from build123d import *
from build123d.topology import SkipClean

# Parameters (mm, degrees)
SKETCH1_R                = 9.3
SKETCH1_R_2              = 6.15
BOSS_EXTRUDE1_DEPTH      = 12.2
BOSS_EXTRUDE2_START      = 4
SKETCH2_R                = 9.3
SKETCH2_R_2              = 6.15
BOSS_EXTRUDE2_DEPTH      = 12
BOSS_EXTRUDE3_DEPTH      = 10
BOSS_EXTRUDE3_DEPTH_BACK = 6
SKETCH3_R                = 13.3
SKETCH3_R_2              = 12.3
SKETCH4_R                = 13.3
SKETCH4_R_2              = 9.3
BOSS_EXTRUDE4_DEPTH      = 2
CUT_EXTRUDE1_START       = -6
CUT_EXTRUDE1_DEPTH       = 6
CUT_EXTRUDE2_START       = -16
CUT_EXTRUDE2_DEPTH       = 6
BOSS_EXTRUDE5_START      = 4
SKETCH7_R                = 9.3
BOSS_EXTRUDE5_DEPTH      = 4
BOSS_EXTRUDE6_START      = 2
SKETCH8_R                = 13.3
SKETCH8_R_2              = 9.3
BOSS_EXTRUDE6_DEPTH      = 2
SKETCH9_R                = 9.3
SKETCH9_R_2              = 6.15
BOSS_EXTRUDE7_DEPTH      = 4
FILLET1_R                = 4
FILLET2_R                = 4
FILLET3_R                = 2
FILLET4_R                = 2
FILLET5_R                = 2


# Some blends are built 0.0001 mm under size
with BuildPart() as part:
    # Sketch1 → Boss-Extrude1 (new body)
    with BuildSketch(Plane(origin=(0, 0, 0), x_dir=(1, 0, 0), z_dir=(0, 1, 0))):
        with Locations(Location((0, 0, 0), (0, 0, 270))):
            Circle(SKETCH1_R)
        with Locations(Location((0, 0, 0), (0, 0, 270))):
            Circle(SKETCH1_R_2, mode=Mode.SUBTRACT)
    extrude(amount=BOSS_EXTRUDE1_DEPTH)

    # Sketch5 → Cut-Extrude1 (cut)
    with BuildSketch(Plane.XZ.offset(CUT_EXTRUDE1_START)):
        with BuildLine():
            Line((9.01494402, 2.284903569), (5.709791212, 2.284903569))
            ThreePointArc((5.709791212, 2.284903569), (6.038945105, 1.163461226), (6.15, 0))
            ThreePointArc((6.15, 0), (6.088696755, -0.866182327), (5.906009163, -1.715096431))
            Line((5.906009163, -1.715096431), (9.140483807, -1.715096431))
            ThreePointArc((9.140483807, -1.715096431), (9.260035081, -0.861249265), (9.3, 0))
            ThreePointArc((9.3, 0), (9.228460852, 1.151308085), (9.01494402, 2.284903569))
        make_face()
        with BuildLine():
            ThreePointArc((2, -5.815711478), (0, -6.15), (-2, -5.815711478))
            Line((-2, -5.815711478), (-2, -9.082400564))
            ThreePointArc((-2, -9.082400564), (0, -9.3), (2, -9.082400564))
            Line((2, -9.082400564), (2, -5.815711478))
        make_face()
        with BuildLine():
            ThreePointArc((-5.815711478, -2), (-6.15, 0), (-5.815711478, 2))
            Line((-5.815711478, 2), (-9.082400564, 2))
            ThreePointArc((-9.082400564, 2), (-9.3, 0), (-9.082400564, -2))
            Line((-9.082400564, -2), (-5.815711478, -2))
        make_face()
        with BuildLine():
            ThreePointArc((-2, 5.815711478), (0, 6.15), (2, 5.815711478))
            Line((2, 5.815711478), (2, 9.082400564))
            ThreePointArc((2, 9.082400564), (0, 9.3), (-2, 9.082400564))
            Line((-2, 9.082400564), (-2, 5.815711478))
        make_face()
    extrude(amount=-CUT_EXTRUDE1_DEPTH, mode=Mode.SUBTRACT)



with BuildPart() as body_2:
    # Sketch2 → Boss-Extrude2 (new body)
    with BuildSketch(Plane(origin=(0, 12.2, 0), x_dir=(1, 0, 0), z_dir=(0, 1, 0)).offset(BOSS_EXTRUDE2_START)):
        with Locations(Location((0, 0, 0), (0, 0, 270))):
            Circle(SKETCH2_R)
        with Locations(Location((0, 0, 0), (0, 0, 270))):
            Circle(SKETCH2_R_2, mode=Mode.SUBTRACT)
    extrude(amount=BOSS_EXTRUDE2_DEPTH)



with BuildPart() as body_3:
    # Sketch3 → Boss-Extrude3 (new, two sides: drawn at the far end of the back side and taken through both)
    with BuildSketch(Plane(origin=(0, 12.2, 0), x_dir=(1, 0, 0), z_dir=(0, 1, 0)).offset(-BOSS_EXTRUDE3_DEPTH_BACK)):
        with Locations(Location((0, 0, 0), (0, 0, 270))):
            Circle(SKETCH3_R)
        with Locations(Location((0, 0, 0), (0, 0, 270))):
            Circle(SKETCH3_R_2, mode=Mode.SUBTRACT)
    extrude(amount=BOSS_EXTRUDE3_DEPTH + BOSS_EXTRUDE3_DEPTH_BACK)


with BuildPart() as body_2_1:
    add(body_2.part)

    add(body_3.part)  # Boss-Extrude4 merges body 3
    # Sketch4 → Boss-Extrude4 (add)
    with BuildSketch(Plane(origin=(0, 22.2, 0), x_dir=(1, 0, 0), z_dir=(0, 1, 0))):
        with Locations(Location((0, 0, 0), (0, 0, 270))):
            Circle(SKETCH4_R)
        with Locations(Location((0, 0, 0), (0, 0, 270))):
            Circle(SKETCH4_R_2, mode=Mode.SUBTRACT)
    extrude(amount=BOSS_EXTRUDE4_DEPTH)

    # Sketch6 → Cut-Extrude2 (cut)
    with BuildSketch(Plane.XZ.offset(CUT_EXTRUDE2_START)):
        with BuildLine():
            ThreePointArc((2, -5.815711478), (0, -6.15), (-2, -5.815711478))
            Line((-2, -5.815711478), (-2, -9.082400564))
            ThreePointArc((-2, -9.082400564), (0, -9.3), (2, -9.082400564))
            Line((2, -9.082400564), (2, -5.815711478))
        make_face()
        with BuildLine():
            Line((-9.082400564, -2), (-5.815711478, -2))
            ThreePointArc((-5.815711478, -2), (-6.15, 0), (-5.815711478, 2))
            Line((-5.815711478, 2), (-9.082400564, 2))
            ThreePointArc((-9.082400564, 2), (-9.3, 0), (-9.082400564, -2))
        make_face()
        with BuildLine():
            Line((-2, 9.082400564), (-2, 5.815711478))
            ThreePointArc((-2, 5.815711478), (0, 6.15), (2, 5.815711478))
            Line((2, 5.815711478), (2, 9.082400564))
            ThreePointArc((2, 9.082400564), (0, 9.3), (-2, 9.082400564))
        make_face()
        with BuildLine():
            Line((9.082400564, 2), (5.815711478, 2))
            ThreePointArc((5.815711478, 2), (6.06585219, 1.01387238), (6.15, 0))
            ThreePointArc((6.15, 0), (6.06585219, -1.01387238), (5.815711478, -2))
            Line((5.815711478, -2), (9.082400564, -2))
            ThreePointArc((9.082400564, -2), (9.245440099, -1.005901277), (9.3, 0))
            ThreePointArc((9.3, 0), (9.245440099, 1.005901277), (9.082400564, 2))
        make_face()
    extrude(amount=-CUT_EXTRUDE2_DEPTH, mode=Mode.SUBTRACT)


with BuildPart() as part_1:
    add(part.part)

    add(body_2_1.part)  # Boss-Extrude5 merges body 2
    # Sketch7 → Boss-Extrude5 (add)
    with BuildSketch(Plane.XZ.offset(-16.2).offset(BOSS_EXTRUDE5_START)):
        with Locations(Location((0, 0, 0), (0, 0, 90))):
            Circle(SKETCH7_R)
    extrude(amount=-BOSS_EXTRUDE5_DEPTH)

    # Sketch8 → Boss-Extrude6 (add)
    with BuildSketch(Plane.XZ.offset(-6.2).offset(BOSS_EXTRUDE6_START)):
        with Locations(Location((0, 0, 0), (0, 0, 270))):
            Circle(SKETCH8_R)
        with Locations(Location((0, 0, 0), (0, 0, 282.418681506))):
            Circle(SKETCH8_R_2, mode=Mode.SUBTRACT)
    extrude(amount=-BOSS_EXTRUDE6_DEPTH)

    # Sketch9 → Boss-Extrude7 (add)
    with SkipClean():  # the faces are left unmerged after this step: merging them gives an invalid solid
        with BuildSketch(Plane(origin=(0, 28.2, 0), x_dir=(1, 0, 0), z_dir=(0, 1, 0))):
            with Locations(Location((0, 0, 0), (0, 0, 77.581318494))):
                Circle(SKETCH9_R)
            with Locations(Location((0, 0, 0), (0, 0, 90))):
                Circle(SKETCH9_R_2, mode=Mode.SUBTRACT)
        extrude(amount=BOSS_EXTRUDE7_DEPTH)

    # Fillet1
    fillet1_edges = [part_1.edges().sort_by_distance(p)[0] for p in [
        (0, 4.2, -9.3),
    ]]
    fillet(fillet1_edges, radius=FILLET1_R - 0.0001)  # a hair under: the kernel refuses the full size

    # Fillet2
    fillet2_edges = [part_1.edges().sort_by_distance(p)[0] for p in [
        (0, 24.2, -9.3),
    ]]
    fillet(fillet2_edges, radius=FILLET2_R - 0.0001)  # a hair under: the kernel refuses the full size

    # Fillet3
    fillet3_edges = [part_1.edges().sort_by_distance(p)[0] for p in [
        (-2, 32.2, 9.082400564),
    ]]
    fillet(fillet3_edges, radius=FILLET3_R)

    # Fillet4
    # the kernel refuses this fillet: 2 mm, written as the material it takes off along each edge
    with BuildSketch(Plane(origin=(0, 24.2, 0), x_dir=(0, 0, 1), z_dir=(-1, 0, 0))) as fillet4_piece_1:
        with BuildLine():
            CenterArc((11.3, -1.656883538), FILLET4_R, 0, 70.529454613)
            Line((13.3, -1.656883538), (13.5, -1.656883538))
            Line((13.5, -1.656883538), (13.5, 0))
            Line((13.5, 0), (13.3, 0.2))
            ThreePointArc((13.3, 0.2), (13.2999, 0.2), (12.033308888, 0.417304996))
            Line((12.033308888, 0.417304996), (11.966644444, 0.228742402))
        make_face()
    revolve(axis=Axis((0, 24.2, 0), (0, 1, 0)), mode=Mode.SUBTRACT)

    # Fillet5
    # the kernel refuses this fillet: 2 mm, written as the material it takes off along each edge
    with BuildSketch(Plane(origin=(0, 4.2, 0), x_dir=(0, 0, -1), z_dir=(-1, 0, 0))) as fillet5_piece_1:
        with BuildLine():
            CenterArc((11.3, -1.656883538), FILLET5_R, 0, 70.529454613)
            Line((11.966644444, 0.228742402), (12.033308888, 0.417304996))
            ThreePointArc((12.033308888, 0.417304996), (13.2999, 0.2), (13.3, 0.2))
            Line((13.3, 0.2), (13.5, 0))
            Line((13.5, 0), (13.5, -1.656883538))
            Line((13.5, -1.656883538), (13.3, -1.656883538))
        make_face()
    revolve(axis=Axis((0, 4.2, 0), (0, -1, 0)), mode=Mode.SUBTRACT)


solid = part_1.part
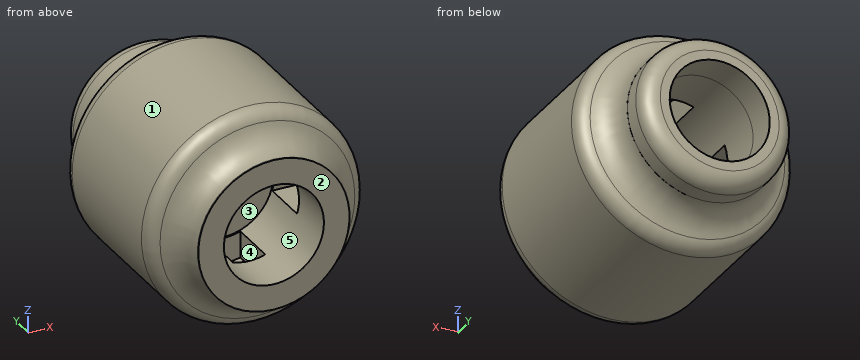
The model under review builds one solid part; all positions refer to its coordinate system, in mm. Face numbers are marked on the shaded views. A direction names the side the tool comes from. Round coordinates to 2 decimals unless told otherwise and drop trailing zeros. Order: outer loops, then holes, each group sorted by start corner. A loop starts at its lowest first (then second) coordinate and runs counter-clockwise, first axis right, second up. Notation, with made-up numbers: (31.5, -12) -> (45.5, -12) arc R20 ccw to (45.5, 16) -> close; hole circle Ø3 at (-13.75, 35). An arc over 180 degrees is marked (long way). Use CSV: the item, a comma, the result in double quotes. Start each with the question number.
(1) Consider section B-B on z = 0. State how many separate pieces and enclosed holes the cut face has, and give its area (3 significant figures).
(2) Insertion check: pin 1 (12 mm diameter, centred on x = 9.5, y = 8, fed in from +Z); pin 2 (1 mm diameter, centred on x = -7.5, y = 19.5, fed in from +Z); pin 3 (2 mm diameter, centred on x = -8.5, y = 6.5, fed in from -Z). Each pin has a flat end and moves straight along its axis. Give the tip position at first contact, or say it passes through.
(3) Consider section A-A on y = 14. Write out the cut boundary in (x, z).
(4) Wall thickness on probe 1 along Y at (x, z) = (7, 0.25); probe 2 along X at (y, z) = (18, 0); probe 3 along X at (y, z) = (16, 8.5): over which ranges is each line inside the solid? List them lowest first. Write a range as from..to.
(5) Mouldability with a two-part tool opening along Z and no side actions: class the marked faces 1, 2 and 3 as pulls with the +Z half, pulls with the -Z half, needs draft (parallel to the pull), parting line crosses it, or undercut.
(6) Tool access review of the marked faces 4 and 5: name each direction out of +Z, -Z, +X, -X, +Y, -Y from which nothing blocks a thin tool from reaching the whole face with its end or side.
Responses:
1,separate pieces,"3"
1,enclosed holes,"0"
1,area,"252 mm²"
2,pin 1,"z = 12.83"
2,pin 2,"z = 11.31"
2,pin 3,"z = -10.98"
3,outline,"circle Ø26.6 at (0, 0); circle Ø18.6 at (0, 0); hole circle Ø24.6 at (0, 0)"
4,probe 1,"0..6, 12..16.2, 22..32.2"
4,probe 2,"-13.3..-12.3, 12.3..13.3"
4,probe 3,"-10.23..-8.89, -3.77..3.77, 8.89..10.23"
5,face 1,"parting line crosses it"
5,face 2,"needs draft"
5,face 3,"undercut"
6,face 4,"none"
6,face 5,"-Y"
